The figure shows three views and two pictorial views of one solid part (mm, origin at its lowest corner). Answer the questions. Round coordinates to 2 decimals unless told otherwise and drop trailing zeros. Order: outer loops, then holes, each group sorted by start corner. A loop starts at its lowest first (then second) coordinate and runs counter-clockwise, first axis right, second up.
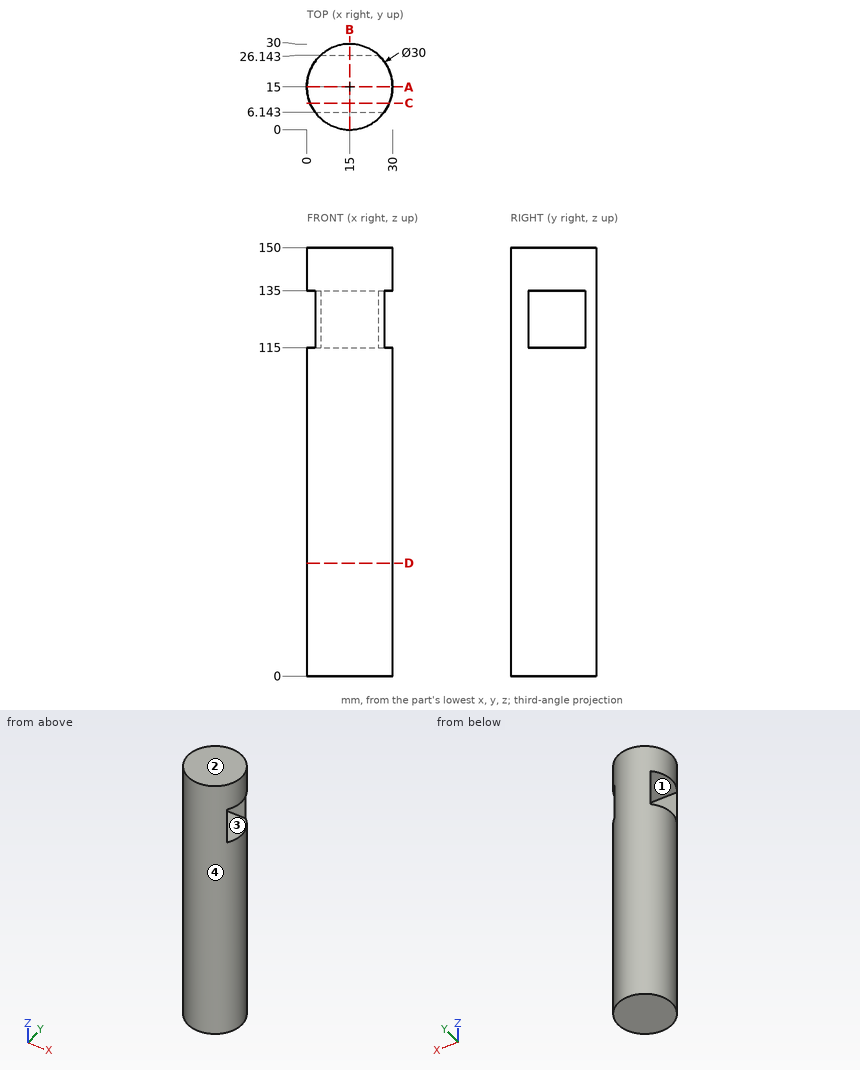
Item 1: Find section D-D (z = 39.5). Write down the section's boundary in (x, y), plus the area to 3 significant figures.
Item 2: Find section A-A (y = 15). Write down the section's boundary in (x, z), plus the area to 3 significant figures.
Item 3: For a pull along Y with two mould halves and no side action, classify the marked faces 1, 2, 3 and 4 as released by +Y, released by -Y, zero draft, split by the parting line, or undercut.
Item 4: Find section B-B (x = 15). Write down the section's boundary in (y, z), plus the area to 3 significant figures.
Item 5: Find section C-C (y = 9.25). Write down the section's boundary in (x, z) (1 decimal), plus the area to 3 significant figures.
Item 6: Find the intervals of material crossed by line 1 along Z through (x, y) = (7, 7); line 2 along Y through (x, z) = (5.25, 130) (1 decimal); line 3 along X through (y, z) = (8.25, 104) (1 decimal), in increasing order.
Item 7: Given pin 1 (1.5 mm diameter, centred on y = 22.5, z = 106, fed in from +X) (1 decimal); pin 2 (6 mm diameter, centred on x = 7, z = 102.5, fed in from -Y); pin 3 (10 mm diameter, centred on y = 23.5, z = 93, fed in from +X), each flat-ended and moving along its own axis, determine where each tip first touches the part or whether it passes through.
Model answer:
1. outline: circle Ø30 at (15, 15)
1. area: 707 mm2
2. outline: (0, 0) - (30, 0) - (30, 115) - (0, 115) - close; (0, 135) - (30, 135) - (30, 150) - (0, 150) - close
2. area: 3,900 mm2
3. face 1: undercut
3. face 2: zero draft
3. face 3: undercut
3. face 4: split by the parting line
4. outline: (0, 0) - (30, 0) - (30, 150) - (0, 150) - close; hole (6.14, 115) - (26.14, 115) - (26.14, 135) - (6.14, 135) - close
4. area: 4,100 mm2
5. outline: (1.1, 0) - (28.9, 0) - (28.9, 115) - (1.1, 115) - close; (1.1, 135) - (28.9, 135) - (28.9, 150) - (1.1, 150) - close
5. area: 3,600 mm2
6. line 1: z = 0 to 115, 135 to 150
6. line 2: y = 3.6 to 6.1, 26.1 to 26.4
6. line 3: x = 1.6 to 28.4
7. pin 1: stops at x = 28.4
7. pin 2: stops at y = 0.86
7. pin 3: stops at x = 29.59
